Can you work these out from the model? Positions are in its coordinate system, mm. A direction names the side the tool comes from. Coordinates: 2 decimals unless noted, no trailing zeros. Order: outer loops, then holes, each group sorted by start corner. A loop starts at its lowest first (then second) coordinate and runs counter-clockwise, first axis right, second up. Notation, with made-up numbers: M 75.5,43.5 L 123.5,43.5 A15 ccw 123.5,72.5 Z; hole C -39,22 d5. An arc over 180 degrees is marked long. Answer as a JSON object with one key per item and string values.
from build123d import *

# Parameters (mm, degrees)
F0_R      = 3.175
F1_DEPTH  = 4.7625
F2_W      = 4.7625
F2_H      = 50.8
F2_H_2    = 76.2
F2_R      = 3.175
F3_DEPTH  = 127
F4_R      = 3.175
F5_DEPTH  = 4.7625
F6_R      = 3.175
F7_DEPTH  = 25.4
F9_DEPTH  = 25.4
F10_W     = 38.1
F10_H     = 38.1
F10_R     = 3.175
F11_DEPTH = 4.7625
F12_W     = 38.1
F12_H     = 38.1
F12_R     = 3.175
F13_DEPTH = 4.7625
F14_W     = 38.1
F14_H     = 38.1
F14_R     = 3.175
F15_DEPTH = 4.7625
F16_W     = 38.1
F16_H     = 38.1
F16_R     = 3.175
F17_DEPTH = 4.7625


# Not quite as in the source:
# - a length typed as a fraction of an inch, garbled in the dataset ("3 / 203.2 mm" for 3/8 in), is restored


with BuildPart() as f1:
    # F0 (on Front) → F1 (new body)
    with BuildSketch(Plane.XZ):
        Polygon((0, 76.2), (0, 0), (505.0019366858, 0), (533.4, 25.4), (609.6, 25.4), (609.6, 76.2), align=None)
        with Locations((38.1, 38.1)):
            Circle(F0_R, mode=Mode.SUBTRACT)
        with Locations((571.5, 50.8)):
            Circle(F0_R, mode=Mode.SUBTRACT)
    extrude(amount=F1_DEPTH)

    # F2 (on face) → F3 (join)
    with BuildSketch(Plane(origin=(0, 0, 0), x_dir=(-1, 0, 0), z_dir=(0, 1, 0))):
        with Locations((-607.21875, 50.8)):
            Rectangle(F2_W, F2_H)
        with Locations((-502.6206866858, 38.1)):
            Rectangle(F2_W, F2_H_2)
        with Locations((-436.7394366858, 50.8)):
            Circle(F2_R)
        with Locations((-322.4394366858, 50.8)):
            Circle(F2_R)
        with Locations((-2.38125, 38.1)):
            Rectangle(F2_W, F2_H_2)
    extrude(amount=F3_DEPTH)

    # F4 (on face) → F5 (join)
    with BuildSketch(Plane(origin=(0, 127, 0), x_dir=(-1, 0, 0), z_dir=(0, 1, 0))):
        Polygon((0, 76.2), (-609.6, 76.2), (-609.6, 25.4), (-533.4, 25.4), (-505.0019366858, 0), (0, 0), align=None)
        with Locations((-571.5, 50.8)):
            Circle(F4_R, mode=Mode.SUBTRACT)
        with Locations((-38.1, 38.1)):
            Circle(F4_R, mode=Mode.SUBTRACT)
    extrude(amount=F5_DEPTH)

    # F6 (on face) → F7 (cut)
    with BuildSketch(Plane.YZ.offset(609.6)):
        with Locations((63.5, 63.5)):
            Circle(F6_R)
    extrude(amount=-F7_DEPTH, mode=Mode.SUBTRACT)

    # F8 (on face) → F9 (cut)
    with BuildSketch(Plane.YZ.offset(505.0019366858)):
        Polygon((74.4985226281, 76.2), (63.5, 76.2), (63.5, 69.85), align=None)
        Polygon((63.5, 69.85), (63.5, 76.2), (52.5014773719, 76.2), align=None)
    extrude(amount=-F9_DEPTH, mode=Mode.SUBTRACT)

    # F10 (on face) → F11 (join)
    with BuildSketch(Plane(origin=(0, 0, 0), x_dir=(-1, 0, 0), z_dir=(0, 1, 0))):
        with Locations((-38.1, 38.1)):
            Rectangle(F10_W, F10_H)
        with Locations((-38.1, 38.1)):
            Circle(F10_R, mode=Mode.SUBTRACT)
    extrude(amount=F11_DEPTH)

    # F12 (on face) → F13 (join)
    with BuildSketch(Plane(origin=(0, 0, 0), x_dir=(-1, 0, 0), z_dir=(0, 1, 0))):
        with Locations((-571.5, 50.8)):
            Rectangle(F12_W, F12_H)
        with Locations((-571.5, 50.8)):
            Circle(F12_R, mode=Mode.SUBTRACT)
    extrude(amount=F13_DEPTH)

    # F14 (on face) → F15 (join)
    with BuildSketch(Plane(origin=(0, 127, 0), x_dir=(-1, 0, 0), z_dir=(0, 1, 0))):
        with Locations((-38.1, 38.1)):
            Rectangle(F14_W, F14_H)
        with Locations((-38.1, 38.1)):
            Circle(F14_R, mode=Mode.SUBTRACT)
    extrude(amount=-F15_DEPTH)

    # F16 (on face) → F17 (join)
    with BuildSketch(Plane(origin=(0, 127, 0), x_dir=(-1, 0, 0), z_dir=(0, 1, 0))):
        with Locations((-571.5, 50.8)):
            Rectangle(F16_W, F16_H)
        with Locations((-571.5, 50.8)):
            Circle(F16_R, mode=Mode.SUBTRACT)
    extrude(amount=-F17_DEPTH)


solid = f1.part
Item 1: Which directions (+Z, -Z, +X, -X, +Y, -Y) give clear straight access to the entire face, cutting with the end or side of a thin tool? Please do faces 4 (the flat face through (606, 63, 25.4)), 5 (the flat face through (254, 129, 0)), 6 (the flat face through (38, 122.238, 43)).
Answers follow:
{"face 4": "-Z, +X, +Y, -Y", "face 5": "-Z, +X, -X, +Y, -Y", "face 6": "+Z, -Z"}
Item 2: Please list where these lines run through material, in increasing order: line 1 (X direction, y = 123.5, z = 68.5); line 2 (X direction, y = 68, z = 43.5); line 3 (Z direction, x = 608.05, y = 63.5) (3 decimals).
Answers follow:
{"line 1": "x = 0 to 4.76, 500.24 to 505, 552.45 to 590.55, 604.84 to 609.6", "line 2": "x = 0 to 4.76, 500.24 to 505, 604.84 to 609.6", "line 3": "z = 25.4 to 60.325, 66.675 to 76.2"}
Item 3: I'm going to push flat-ended pins straight in: pin 1 (1.4 mm diameter, centred on y = 2, z = 54.5, fed in from -X); pin 2 (8 mm diameter, centred on y = 57.5, z = 18.5, fed in from +X); pin 3 (2.5 mm diameter, centred on x = 35, y = 2, fed in from +Z); pin 4 (1.4 mm diameter, centred on x = 563, y = 125, fed in from +Z). Where does each tip first touch, or does it pass through?
Answers follow:
{"pin 1": "stops at x = 0", "pin 2": "stops at x = 505", "pin 3": "stops at z = 57.15", "pin 4": "stops at z = 69.85"}
Item 4: If we mould it in two halves opening along X, with no side actions, what happens to faces 1 (the flat face through (0, 63, 38)), 2 (the flat face through (249, 0, 39)), 3 (the flat face through (303, 129, 76.2))? For each: pulls with the +X half, pulls with the -X half, needs draft (parallel to the pull), parting line crosses it, or undercut.
Answers follow:
{"face 1": "pulls with the -X half", "face 2": "undercut", "face 3": "needs draft"}
Item 5: I want a section at B-B, the plane y = 35. Give the number of separate pieces and of enclosed holes in the cut face, plus the area to 3 significant figures.
Answers follow:
{"separate pieces": "5", "enclosed holes": "0", "area": "1,030 mm^2"}
Item 6: I want a section at A-A, the plane x = 277. Write out the boundary of the cut face in (y, z), plus the area to 3 significant figures.
Answers follow:
{"outline": "M -4.76,0 L 0,0 L 0,76.2 L -4.76,76.2 Z; M 127,0 L 131.76,0 L 131.76,76.2 L 127,76.2 Z", "area": "726 mm^2"}
